Here's how the part is built. I have some questions about the finished solid (model axes, mm). Coordinates: 2 decimals unless noted, no trailing zeros. Loops run counter-clockwise (first coordinate to the right, second up) from the corner with the lowest first, then second, coordinate; pieces in that order, holes last. Notation, with made-up numbers: (-22.5, -34.5) -> (-12.5, -34.5) arc R16 ccw to (-12.5, -3.5) -> close; hole circle Ø11 at (-26.75, -9.5). An arc over 180 degrees is marked (long way). Use CSV: the item, a comma, the result in double quotes. Start each with the question number.
from build123d import *

# Parameters (mm, degrees)
SKETCH1_R           = 1.6
BOSS_EXTRUDE1_DEPTH = 1.6


with BuildPart() as part:
    # Sketch1 → Boss-Extrude1 (new body)
    with BuildSketch(Plane.XY):
        with BuildLine():
            Line((-13.235657624, 13.611622239), (16.764342376, 13.611622239))
            ThreePointArc((16.764342376, 13.611622239), (18.178555938, 13.025835801), (18.764342376, 11.611622239))
            Line((18.764342376, 11.611622239), (18.764342376, -18.388377761))
            ThreePointArc((18.764342376, -18.388377761), (18.178555938, -19.802591324), (16.764342376, -20.388377761))
            Line((16.764342376, -20.388377761), (-13.235657624, -20.388377761))
            ThreePointArc((-13.235657624, -20.388377761), (-14.649871187, -19.802591324), (-15.235657624, -18.388377761))
            Line((-15.235657624, -18.388377761), (-15.235657624, 11.611622239))
            ThreePointArc((-15.235657624, 11.611622239), (-14.649871187, 13.025835801), (-13.235657624, 13.611622239))
        make_face()
        with Locations((16.764342376, 11.611622239)):
            Circle(SKETCH1_R, mode=Mode.SUBTRACT)
        with Locations(Location((16.764342376, -18.388377761, 0), (0, 0, 180))):
            Circle(SKETCH1_R, mode=Mode.SUBTRACT)
        with Locations(Location((-13.235657624, 11.611622239, 0), (0, 0, 180))):
            Circle(SKETCH1_R, mode=Mode.SUBTRACT)
        with Locations((-13.235657624, -18.388377761)):
            Circle(SKETCH1_R, mode=Mode.SUBTRACT)
    extrude(amount=BOSS_EXTRUDE1_DEPTH)


solid = part.part
1) I want a section at A-A, the plane z = 1.25. Please give me the cut outline in (x, y), plus the area to 3 significant figures.
2) Thinking about a two-plate mould opening in Y: for faces 1 (the face through (2, 13.612, 1)), 2 (the face through (2, -3, 0)), 3 (the face through (-11.71, -17.91, 0.79)), 4 (the face through (-14.63, -19.82, 0.79)), which applies, pulls with the +Y half, pulls with the -Y half, needs draft (parallel to the pull), parting line crosses it, or undercut?
3) I want a section at B-B, the plane y = 11. Please give me the cut outline in (x, z), plus the area to 3 significant figures.
4) Please list where this line runs through material, in increasing order: L1, parallel to X at y = 11, z = 1.5. Write a range as [from, to].
Return value:
1,outline,"(-15.24, -18.39) arc R2 ccw to (-13.24, -20.39) -> (16.76, -20.39) arc R2 ccw to (18.76, -18.39) -> (18.76, 11.61) arc R2 ccw to (16.76, 13.61) -> (-13.24, 13.61) arc R2 ccw to (-15.24, 11.61) -> close; hole circle Ø3.2 at (-13.24, -18.39); hole circle Ø3.2 at (-13.24, 11.61); hole circle Ø3.2 at (16.76, -18.39); hole circle Ø3.2 at (16.76, 11.61)"
1,area,"1,120 mm²"
2,face 1,"pulls with the +Y half"
2,face 2,"needs draft"
2,face 3,"undercut"
2,face 4,"pulls with the -Y half"
3,outline,"(-15.24, 0) -> (-14.71, 0) -> (-14.71, 1.6) -> (-15.24, 1.6) -> close; (-11.76, 0) -> (15.29, 0) -> (15.29, 1.6) -> (-11.76, 1.6) -> close; (18.24, 0) -> (18.76, 0) -> (18.76, 1.6) -> (18.24, 1.6) -> close"
3,area,"44.9 mm²"
4,L1,"x = [-15.24, -14.71], [-11.76, 15.29], [18.24, 18.76]"
